Build history of the part. All positions in model axes, mm. A direction names the side the tool comes from. Give positions to 0.01 mm unless a question says otherwise; leave off trailing zeros. Order: outer loops, then holes, each group sorted by start corner. A loop starts at its lowest first (then second) coordinate and runs counter-clockwise, first axis right, second up. Notation, with made-up numbers: (-30.75, -15) - (-17.75, -15) arc R13 ccw to (-17.75, 1) - close; hole circle Ø8 at (51.5, -1.5). An arc over 180 degrees is marked (long way). One line per item, written item: value.
```python
from build123d import *

# Parameters (mm, degrees)
F1_DEPTH  = 33
F2_W      = 13
F2_H      = 13
F3_DEPTH  = 22.75
F4_W      = 10
F4_H      = 8.67
F5_DEPTH  = 33
F6_W      = 13
F6_H      = 3
F7_DEPTH  = 5
F9_DEPTH  = 6.5
F10_DEPTH = 6.5


with BuildPart() as f1:
    # F0 (on Top) → F1 (new body)
    with BuildSketch(Plane.XY):
        Polygon((-10.25, 13.49995), (-29.225, -13.498744), (29.225, -13.498744), (10.25, 13.49995), align=None)
    extrude(amount=-F1_DEPTH)

    # F2 (on face) → F3 (cut)
    with BuildSketch(Plane(origin=(0, 13.49995, 0), x_dir=(-1, 0, 0), z_dir=(0, 1, 0))):
        with Locations((0, -6.5)):
            Rectangle(F2_W, F2_H)
    extrude(amount=-F3_DEPTH, mode=Mode.SUBTRACT)

    # F4 (on face) → F5 (cut)
    with BuildSketch(Plane.XY):
        with Locations((0.275, -9.163744)):
            Rectangle(F4_W, F4_H)
    extrude(amount=-F5_DEPTH, mode=Mode.SUBTRACT)

    # F6 (on face) → F7 (cut)
    with BuildSketch(Plane.XY.offset(-13)):
        with Locations((0, 9.99995)):
            Rectangle(F6_W, F6_H)
    extrude(amount=-F7_DEPTH, mode=Mode.SUBTRACT)

    # F8 (on Right) → F9 (cut)
    with BuildSketch(Plane.YZ):
        Polygon((-4.83005, -22.918396), (8.49995, -11), (-9.25005, -11), (-9.25005, -22.918396), align=None)
    extrude(amount=-F9_DEPTH, mode=Mode.SUBTRACT)

    # F8 (on Right) → F10 (cut)
    with BuildSketch(Plane.YZ):
        Polygon((-4.83005, -22.918396), (8.49995, -11), (-9.25005, -11), (-9.25005, -22.918396), align=None)
    extrude(amount=F10_DEPTH, mode=Mode.SUBTRACT)


solid = f1.part
```
(1) 3-axis set-ups, long thin cutter, end or side, ignore diameter. For faces 1 (the face through (5.275, -10, -20)), 2 (the face through (-6.5, 2, -9)), 3 (the face through (0, 13.5, -20)): which of +Z, -Z, +X, -X, +Y, -Y reach the whole face in a straight line?
Completed:
face 1: +Z, -Z, -Y
face 2: +Z
face 3: +Z, -Z, +X, -X, +Y
(2) Pull direction Y, two halves, no side cores. Call faces 4 (the face through (0, 7, -13)), 5 (the face through (0, -4.829, -28)), 6 (the face through (-6, -9.25, -11)), 7 (the face through (-6, -7, -22.918)): +Y half, -Y half, draft (parallel to the pull), parting line (faces both ways), or undercut.
Completed:
face 4: draft
face 5: -Y half
face 6: undercut
face 7: undercut
(3) Pin check, flat tips, straight feed: P1, Ø1.1, axis at x = -0.5, y = 7.5, coming from the +Z side; P2, Ø8, axis at y = 3, z = -12, coming from the -X side; P3, Ø0.9, axis at x = 1.5, y = 10, coming from the +Z side; P4, Ø10, axis at x = -1, z = -4, coming from the -Y side. Stop position of each tip, or through.
Completed:
P1: z = -13
P2: x = -20.44
P3: z = -18
P4: y = -13.5
(4) Drill centre lines: line 1 (Z direction, x = 5.5, y = 8.25); line 2 (Y direction, x = -3, z = -25); line 3 (X direction, y = -4.25, z = -18). Where is each one in solid material? Low to high.
Completed:
line 1: -33 to -13
line 2: -4.83 to 13.5
line 3: -22.72 to -6.5, 6.5 to 22.72
(5) Slice it at D-D, the plane z = -29. Give the cut face in (x, y) (3 decimals), and give its area (3 significant figures).
Completed:
outline: (-29.225, -13.499) - (-4.725, -13.499) - (-4.725, -4.829) - (5.275, -4.829) - (5.275, -13.499) - (29.225, -13.499) - (10.25, 13.5) - (-10.25, 13.5) - close
area: 979 mm²
(6) Slice it at C-C, the plane x = 4. Give the cut face in (y, z), and give its area (3 significant figures).
Completed:
outline: (-4.83, -33) - (13.5, -33) - (13.5, -13) - (11.5, -13) - (11.5, -18) - (8.5, -18) - (8.5, -13) - (6.26, -13) - (-4.83, -22.92) - close
area: 297 mm²
(7) Slice it at B-B, the plane y = -6.5. Give the cut face in (x, z) (3 decimals).
Completed:
outline: (-24.306, -33) - (-4.725, -33) - (-4.725, -22.918) - (-6.5, -22.918) - (-6.5, 0) - (-24.306, 0) - close; (5.275, -33) - (24.306, -33) - (24.306, 0) - (6.5, 0) - (6.5, -22.918) - (5.275, -22.918) - close
(8) Slice it at A-A, the plane z = -9.5. Give the cut face in (x, y) (3 decimals).
Completed:
outline: (-29.225, -13.499) - (-4.725, -13.499) - (-4.725, -9.25) - (-6.5, -9.25) - (-6.5, 13.5) - (-10.25, 13.5) - close; (5.275, -13.499) - (29.225, -13.499) - (10.25, 13.5) - (6.5, 13.5) - (6.5, -9.25) - (5.275, -9.25) - close
